Source: CAD feature listing. Evaluate the final solid. Frame: model axes, mm. Face numbers are marked on the shaded views. A direction names the side the tool comes from. Give positions to 0.01 mm unless a question says otherwise; leave off trailing zeros. Order: outer loops, then holes, each group sorted by start corner. A loop starts at its lowest first (then second) coordinate and runs counter-clockwise, first axis right, second up. Notation, with made-up numbers: M -29,61.25 L -4,61.25 A16 ccw -4,75.25 Z; hole C 74.25,34 d11. An arc over 180 degrees is marked long. Answer as a JSON object with one key per item and string values. Group by question number.
1. Pull-direction query (Z, two-part tool) for the marked faces 6, 7 and 8; classes: +Z half, -Z half, draft (parallel to the pull), parting line (faces both ways), or undercut.
2. Section query C-C (z = 7.25). Output: boundary loops of the cut face in (x, y).
3. Section query A-A (z = 0). Output: boundary loops of the cut face in (x, y).
4. Section query B-B (y = -4.5). Count the separate pieces of the cut face and the enclosed holes in it, plus the area to 3 significant figures.
5. Material intervals for L1, parallel to Z at x = -6, y = -7.5; L2, parallel to Z at x = 0, y = 0.5; L3, parallel to X at y = -2.25, z = -5.25, sorted ascending. Write a range as [from, to].
6. Pin query (flat end, axial travel): P1, Ø4, axis at y = -3.5, z = -5, coming from the -X side; P2, Ø6, axis at y = -5, z = -3, coming from the +X side; P3, Ø6, axis at y = -7.5, z = 6, coming from the +X side; P4, Ø1.2, axis at x = 0, z = 0, coming from the -Y side. Return the tip coordinate at first contact, or that it passes through.
7. Set-up query: the marked faces 1, 2, 3, 4 and 5. Return all of +Z, -Z, +X, -X, +Y, -Y with unobstructed straight access to the full face (end or side cutting, diameter ignored); none if empty.
Autodesk Inventor part; units mm, degrees
ref_plane "YZ Plane" through (0, 0, 0) normal (1, 0, 0) x (0, 1, 0)
ref_plane "XZ Plane" through (0, 0, 0) normal (0, 1, 0) x (-1, 0, 0)
ref_plane "XY Plane" through (0, 0, 0) normal (0, 0, 1) x (1, 0, 0)
sketch "Sketch1" plane through (0, 0, 0) normal (0, 1, 0) x (-1, 0, 0)
  circle A0 centre (0, 0) radius 10
  circle A1 centre (0, 0) radius 1
  dimension "d0" = 20
  dimension "d1" = 2
extrude "Extrusion1" add sketch "Sketch1" along normal blind 1.5875
sketch "Sketch2" plane through (0, 0, 0) normal (0, -1, 0) x (1, 0, 0)
  circle A0 centre (0, 0) radius 1
  circle A1 centre (0, 0) radius 2.54
  dimension "d4" = 5.08
extrude "Extrusion2" add sketch "Sketch2" along normal blind 5.08
sketch "Sketch3" plane through (0, 0, 0) normal (0, -1, 0) x (1, 0, 0)
  arc A0 (0.2215, -4.3806) -> (1.0574, -9.2715) centre (11.9577, -4.8916) ccw
  arc A1 (-0.6328, -4.3141) -> (0.1422, -9.6491) centre (9.9382, -5.5021) ccw
  arc A2 (0.1422, -9.6491) -> (1.0574, -9.2715) centre (0.5981, -9.4561) ccw
  arc A3 (0.2215, -4.3806) -> (-0.6328, -4.3141) centre (-0.2068, -4.362) ccw
  point P0 (0, 0)
  dimension "d7" = 1
extrude "Extrusion3" add sketch "Sketch3" along normal blind 10.16
pattern_circular "Circular Pattern1" count 10 over 360 about axis through (0, 0, 0) along (0, 1, 0) of "Extrusion3"
chamfer "Chamfer1" distance 1.27 angle 45 1 edges at (-2.54, -5.08, 0)
properties part number "Fan Blade"
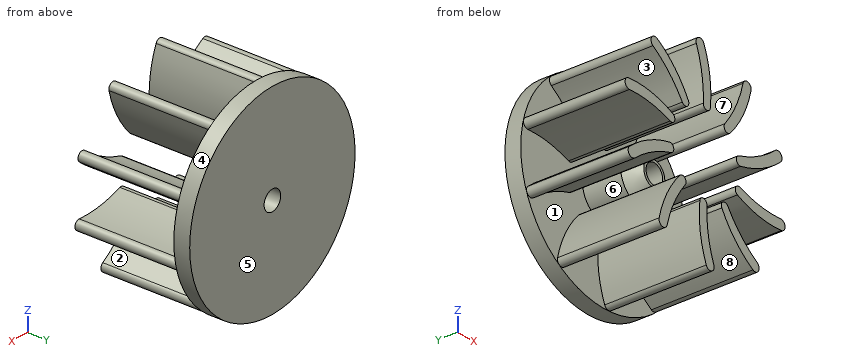
Answer sheet:
{
 "1": {"face 6": "undercut", "face 7": "+Z half", "face 8": "-Z half"},
 "2": {"outline": "M -6.89,0 L -6.53,0 L -6.53,-10.16 L -5.07,-10.16 L -5.07,0 L -0.45,0 L -0.45,-10.16 L 0.55,-10.16 L 0.55,0 L 4.34,0 L 4.34,-10.16 L 5.39,-10.16 L 5.39,0 L 6.89,0 L 6.89,1.59 L -6.89,1.59 Z"},
 "3": {"outline": "M -10,0 L -2.54,0 L -2.54,-3.81 L -1.27,-5.08 L -1,-5.08 L -1,1.59 L -10,1.59 Z; M 1,-5.08 L 1.27,-5.08 L 2.54,-3.81 L 2.54,0 L 10,0 L 10,1.59 L 1,1.59 Z"},
 "4": {"separate pieces": "11", "enclosed holes": "1", "area": "64.4 mm^2"},
 "5": {"L1": "[-2.27, -1.23], [1.65, 2.63], [6.68, 7.79]", "L2": "[-10, -1], [1, 10]", "L3": "[-4.56, -3.45], [-0.7, 0.22], [2.96, 4.26]"},
 "6": {"P1": "x = -9.3", "P2": "x = 9.67", "P3": "x = 9.3", "P4": "through"},
 "7": {"face 1": "-Y", "face 2": "+X, -Y", "face 3": "-X, -Y", "face 4": "+Y, -Y", "face 5": "+Z, -Z, +X, -X, +Y"}
}
